Geometry: see drawing. Coordinates: mm, zero at the bounding-box minimum. A direction names the side the tool comes from. Coordinates: 2 decimals unless noted, no trailing zeros. Write each loop counter-clockwise with the first axis right and the second up, starting at its lowest first coordinate (ties: lowest second). Pieces come first, ordered by that corner, then holes. Notation, with made-up numbers: (24, 86) -> (44, 86) arc R23 ccw to (44, 115) -> close; hole circle Ø3 at (27, 25.25). An arc over 180 degrees is marked (long way). Use one line per item in the form item = value. Start each with the question number.
(1) Ray query, line 1 along X through (y, z) = (9.5, 11.5); line 2 along Y through (x, z) = (12, 11.25); line 3 along X through (y, z) = (24, 3.25). Return the intervals inside material, ascending.
(2) Set-up query: the marked faces 4, 5, 6 and 7. Return all of +Z, -Z, +X, -X, +Y, -Y with unobstructed straight access to the full face (end or side cutting, diameter ignored); none if empty.
(3) Pull-direction query (X, two-part tool) for the marked faces 1, 2 and 3; classes: released by +X, released by -X, zero draft, split by the parting line, or undercut.
(4) Cut plane C-C on z = 12.5. Return the cut outline in (x, y).
(5) First-contact query: pin 1 (4.5 mm diameter, centred on x = 4, z = 7, fed in from -Y); pin 2 (1 mm diameter, centred on y = 19, z = 13.5, fed in from +X); pin 3 (4.5 mm diameter, centred on x = 145, z = 4, fed in from +Y). Flat tips, straight axial feed; report the tip coordinate or a pass-through.
(6) Cut plane A-A on y = 10. Return the cut outline in (x, z).
(7) Cut plane B-B on x = 12.5. Return the cut outline in (y, z), plus the area to 3 significant figures.
(8) Cut plane D-D on y = 19.5. Return the cut outline in (x, z).
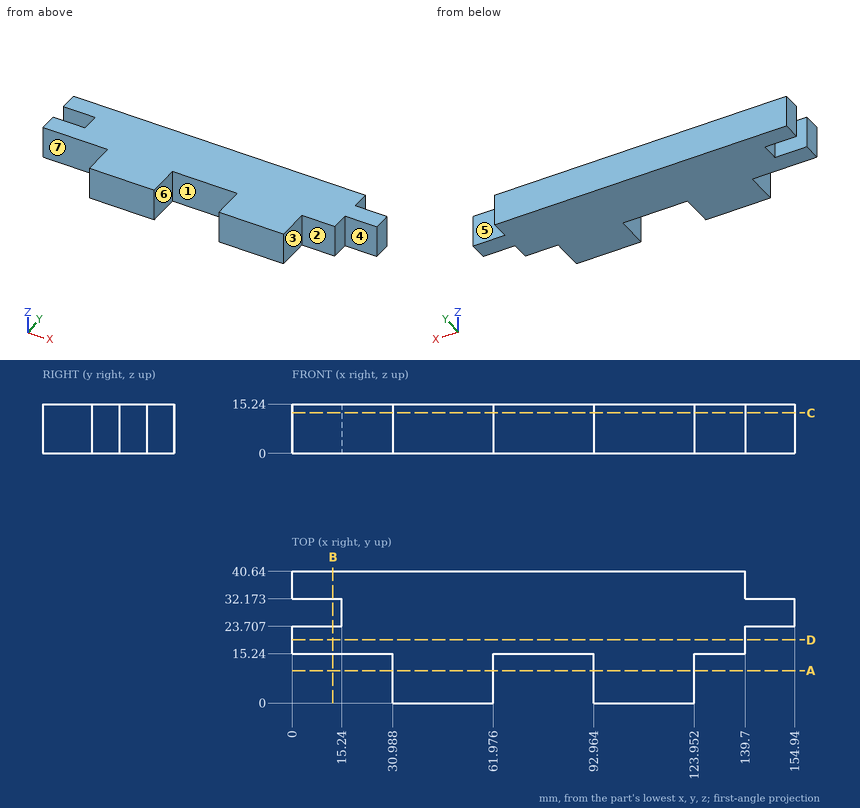
Values:
q1.line_1 = 30.99 to 61.98, 92.96 to 123.95
q1.line_2 = 15.24 to 23.71, 32.17 to 40.64
q1.line_3 = 15.24 to 154.94
q2.face_4 = +Z, -Z, +X, -Y
q2.face_5 = +Z, -Z, +X, +Y
q2.face_6 = +Z, -Z, -Y
q2.face_7 = +Z, -Z, -X, -Y
q3.face_1 = undercut
q3.face_2 = zero draft
q3.face_3 = released by +X
q4.outline = (0, 15.24) -> (30.99, 15.24) -> (30.99, 0) -> (61.98, 0) -> (61.98, 15.24) -> (92.96, 15.24) -> (92.96, 0) -> (123.95, 0) -> (123.95, 15.24) -> (139.7, 15.24) -> (139.7, 23.71) -> (154.94, 23.71) -> (154.94, 32.17) -> (139.7, 32.17) -> (139.7, 40.64) -> (0, 40.64) -> (0, 32.17) -> (15.24, 32.17) -> (15.24, 23.71) -> (0, 23.71) -> close
q5.pin_1 = 15.24
q5.pin_2 = 139.7
q5.pin_3 = 32.17
q6.outline = (30.99, 0) -> (61.98, 0) -> (61.98, 15.24) -> (30.99, 15.24) -> close; (92.96, 0) -> (123.95, 0) -> (123.95, 15.24) -> (92.96, 15.24) -> close
q7.outline = (15.24, 0) -> (23.71, 0) -> (23.71, 15.24) -> (15.24, 15.24) -> close; (32.17, 0) -> (40.64, 0) -> (40.64, 15.24) -> (32.17, 15.24) -> close
q7.area = 258 mm2
q8.outline = (0, 0) -> (139.7, 0) -> (139.7, 15.24) -> (0, 15.24) -> close
